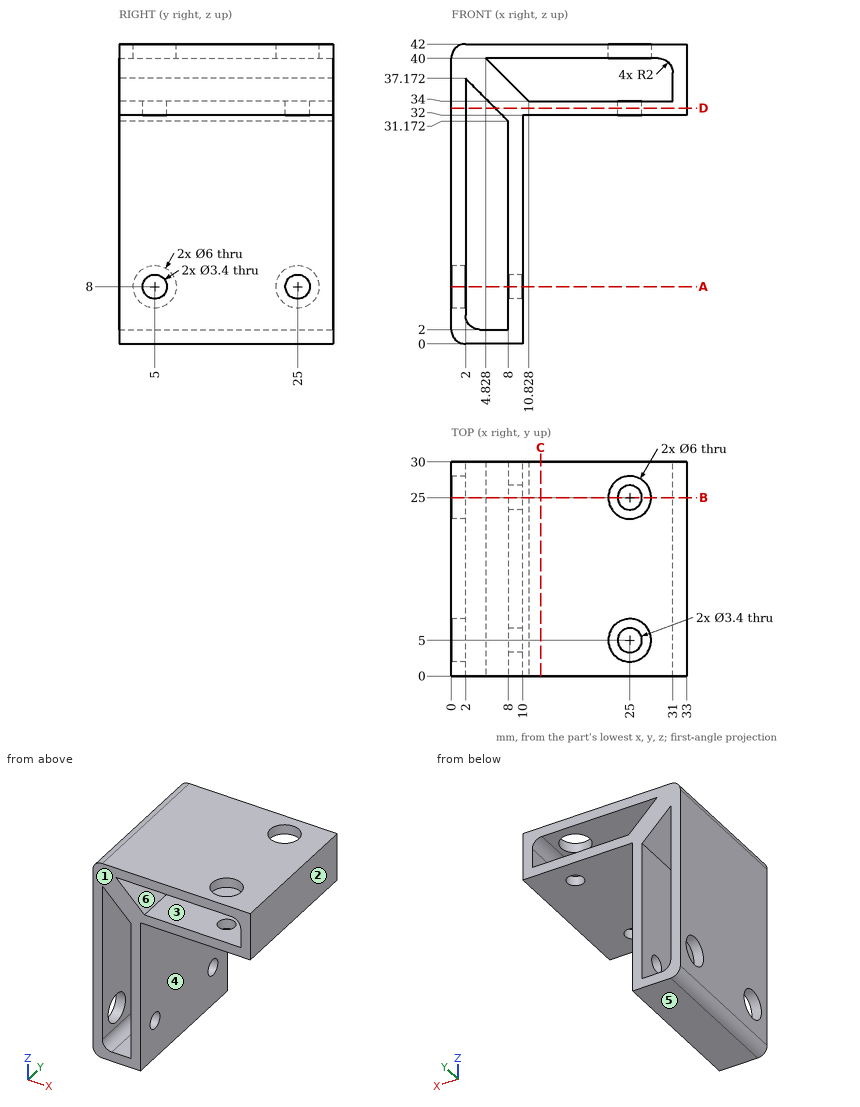
Input: dimensioned drawing with shaded views. Units: mm. Origin: part minimum x, y, z. A direction names the side the tool comes from. Coordinates: 2 decimals unless noted, no trailing zeros. Order: outer loops, then holes, each group sorted by start corner. A loop starts at its lowest first (then second) coordinate and runs counter-clockwise, first axis right, second up. Notation, with made-up numbers: (11, -30.75) - (43, -30.75) arc R20 ccw to (43, 8.25) - close; hole circle Ø11 at (67.25, 11). An arc over 180 degrees is marked (long way). One line per item, written item: value.
1) Cut plane A-A on z = 8. Output: boundary loops of the cut face in (x, y).
Computed values:
outline: (0, 0) - (2, 0) - (2, 2) - (0, 2) - close; (0, 8) - (2, 8) - (2, 22) - (0, 22) - close; (0, 28) - (2, 28) - (2, 30) - (0, 30) - close; (8, 0) - (10, 0) - (10, 3.3) - (8, 3.3) - close; (8, 6.7) - (10, 6.7) - (10, 23.3) - (8, 23.3) - close; (8, 26.7) - (10, 26.7) - (10, 30) - (8, 30) - close
2) Cut plane D-D on z = 33. Output: boundary loops of the cut face in (x, y).
Computed values:
outline: (0, 0) - (2, 0) - (2, 30) - (0, 30) - close; (6.17, 0) - (33, 0) - (33, 30) - (6.17, 30) - close; hole circle Ø3.4 at (25, 5); hole circle Ø3.4 at (25, 25)
3) Cut plane C-C on x = 12.5. Output: boundary loops of the cut face in (y, z).
Computed values:
outline: (0, 32) - (30, 32) - (30, 34) - (0, 34) - close; (0, 40) - (30, 40) - (30, 42) - (0, 42) - close
4) Contact query for flat-ended pins moving along their axis: pin 1 (9 mm diameter, centred on y = 10, z = 18.5, fed in from +X); pin 2 (1.5 mm diameter, centred on x = 15, y = 6, fed in from -Z); pin 3 (4 mm diameter, centred on x = 25, y = 25, fed in from +Z). Output: stop coordinate, or through.
Computed values:
pin 1: stops at x = 10
pin 2: stops at z = 32
pin 3: stops at z = 34
5) Cut plane B-B on y = 25. State how many separate pieces and enclosed holes the cut face has.
Computed values:
separate pieces: 3
enclosed holes: 0
6) Reachability of the marked faces 4, 5 and 6 from +Z, -Z, +X, -X, +Y, -Y: full face, straight path, thin tool, end or side. Return the list, or none.
Computed values:
face 4: -Z, +X, +Y, -Y
face 5: -Z, +X, -X, +Y, -Y
face 6: +Y, -Y
7) Mould query, pull axis X, two halves, no side actions, for the marked faces 1, 2 and 3. Classes: released by +X, released by -X, zero draft, split by the parting line, or undercut.
Computed values:
face 1: zero draft
face 2: released by +X
face 3: undercut
8) Ray query, line 1 (Y direction, x = 25, z = 41.4); line 2 (Y direction, x = 9, z = 8); line 3 (X direction, y = 11.5, z = 11). Return the intervals inside material, ascending. Write a range as [from, to].
Computed values:
line 1: y = [0, 2], [8, 22], [28, 30]
line 2: y = [0, 3.3], [6.7, 23.3], [26.7, 30]
line 3: x = [0, 2], [8, 10]
